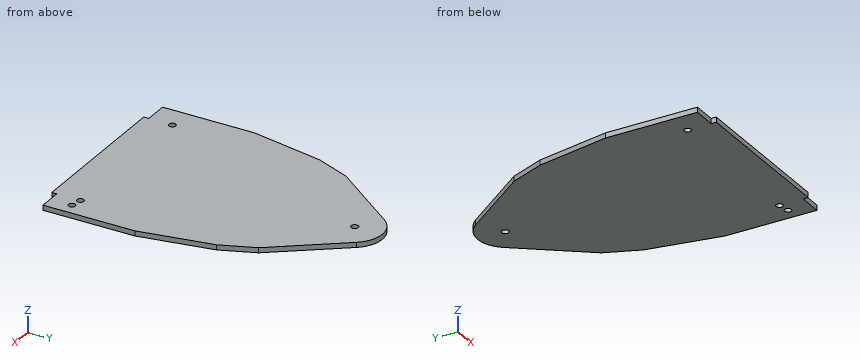
from build123d import *

# Parameters (mm, degrees)
F0_W     = 30
F0_H     = 20
F0_R     = 2.25
F1_DEPTH = 3.2
F2_R     = 2.15
F3_DEPTH = 54
F4_W     = 100
F4_H     = 3.2
F5_DEPTH = 3.2


with BuildPart() as f1:
    # F0 (on Top) → F1 (new body)
    with BuildSketch(Plane.XY):
        Polygon((-65, -75), (65, -75), (65, 75), (30, 75), (15, 75), (-15, 75), (-30, 75), (-65, 75), align=None)
        Polygon((15, 75), (30, 75), (15, 95), align=None)
        Polygon((-15, 95), (-30, 75), (-15, 75), align=None)
        with Locations((0, 85)):
            Rectangle(F0_W, F0_H)
        with Locations((0, 85)):
            Circle(F0_R, mode=Mode.SUBTRACT)
        with BuildLine():
            Line((-15, 95), (15, 95))
            ThreePointArc((15, 95), (0, 102.5), (-15, 95))
        make_face()
    extrude(amount=F1_DEPTH)

    # F2 (on Top) → F3 (cut)
    with BuildSketch(Plane.XY):
        with Locations((-50, -60)):
            Circle(F2_R)
        with Locations((50, -60)):
            Circle(F2_R)
        Polygon((-30, 75), (-65, 75), (-65, 28.3333333333), (-47.5, 51.6666666667), align=None)
        Polygon((-47.5, 51.6666666667), (-65, 28.3333333333), (-65, 8.3333333333), (-56.25, 30), align=None)
        Polygon((-56.25, 30), (-65, 8.3333333333), (-65, -16.6666666667), align=None)
        Polygon((65, 8.3333333333), (65, 75), (30, 75), (47.5, 51.6666666667), (56.25, 30), align=None)
        Polygon((65, -16.6666666667), (65, 8.3333333333), (56.25, 30), align=None)
        with Locations((57, -61.25)):
            Circle(F2_R)
    extrude(amount=F3_DEPTH, mode=Mode.SUBTRACT)

    # F4 (on Top) → F5 (join)
    with BuildSketch(Plane.XY):
        with Locations((0, -76.6)):
            Rectangle(F4_W, F4_H)
    extrude(amount=F5_DEPTH)


solid = f1.part
Geometry: final body of the model. Coordinates: model frame, mm. Give positions to 0.01 mm unless a question says otherwise; leave off trailing zeros. Order: outer loops, then holes, each group sorted by start corner. A loop starts at its lowest first (then second) coordinate and runs counter-clockwise, first axis right, second up. Notation, with made-up numbers: (23, 22) -> (32, 22) arc R19 cw to (32, 51) -> close; hole circle Ø2 at (73, -22.5). An arc over 180 degrees is marked (long way). Put each result on its own line as item: value.
Q1. Section A-A, the plane y = 85. Return loops of the section in (x, z), then the cut area to 3 significant figures.
Here are the results:
outline: (-22.5, 0) -> (-2.25, 0) -> (-2.25, 3.2) -> (-22.5, 3.2) -> close; (2.25, 0) -> (22.5, 0) -> (22.5, 3.2) -> (2.25, 3.2) -> close
area: 130 mm^2
Q2. Section D-D, the plane x = 28.5. Return loops of the section in (y, z), then the cut area to 3 significant figures.
Here are the results:
outline: (-78.2, 0) -> (77, 0) -> (77, 3.2) -> (-78.2, 3.2) -> close
area: 497 mm^2
Q3. Material intervals for L1, parallel to Y at x = 0, z = 1.2; L2, parallel to X at y = -61, z = 1.15; L3, parallel to X at y = -61.25, z = 1.5, sorted ascending.
Here are the results:
L1: y = -78.2 to 82.75, 87.25 to 102.5
L2: x = -65 to -51.9, -48.1 to 48.1, 51.9 to 54.86, 59.14 to 65
L3: x = -65 to -51.75, -48.25 to 48.25, 51.75 to 54.85, 59.15 to 65
Q4. Section C-C, the plane z = 0.7. Return loops of the section in (x, y).
Here are the results:
outline: (-65, -75) -> (-50, -75) -> (-50, -78.2) -> (50, -78.2) -> (50, -75) -> (65, -75) -> (65, -16.67) -> (56.25, 30) -> (47.5, 51.67) -> (15, 95) arc R18.75 ccw to (-15, 95) -> (-47.5, 51.67) -> (-56.25, 30) -> (-65, -16.67) -> close; hole circle Ø4.3 at (-50, -60); hole circle Ø4.5 at (0, 85); hole circle Ø4.3 at (50, -60); hole circle Ø4.3 at (57, -61.25)
Q5. Pin query (flat end, axial travel): pin 1 (1 mm diameter, centred on x = 57.5, z = 2, fed in from -Y); pin 2 (1.5 mm diameter, centred on x = 8, z = 0.5, fed in from +Y). Return the tip coordinate at first contact, or that it passes through.
Here are the results:
pin 1: stops at y = -75
pin 2: stops at y = 101.04
Q6. Section B-B, the plane x = 0. Return loops of the section in (y, z).
Here are the results:
outline: (-78.2, 0) -> (82.75, 0) -> (82.75, 3.2) -> (-78.2, 3.2) -> close; (87.25, 0) -> (102.5, 0) -> (102.5, 3.2) -> (87.25, 3.2) -> close
